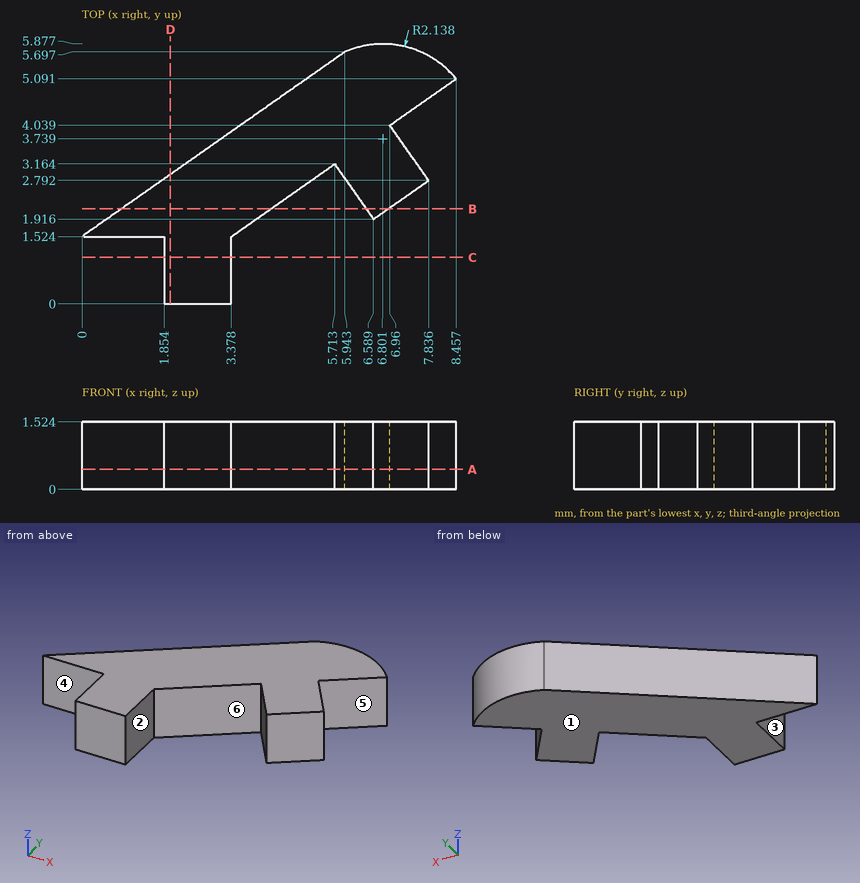
Could you check a few things on this drawing? It's one solid part, dimensions in mm from its lowest x, y, z. A direction names the side the tool comes from. Coordinates: 2 decimals unless noted, no trailing zeros. Order: outer loops, then holes, each group sorted by start corner. A loop starts at its lowest first (then second) coordinate and runs counter-clockwise, first axis right, second up. Notation, with made-up numbers: M -25.5,16 L -12.5,16 A26 ccw -12.5,36 Z; hole C 9.25,-6 d4. An arc over 180 degrees is marked long. Use a Markdown table: item, result. Add a question column.
Q1. I'm going to push flat-ended pins straight in: pin 1 (0.5 mm diameter, centred on x = 1, z = 0.5, fed in from -Y); pin 2 (0.8 mm diameter, centred on y = 1, z = 1, fed in from +X). Where does each tip first touch, or does it pass through?
Q2. I want a section at C-C on y = 1.05. List the corners of the cut face in (x, z) for me.
Q3. We'd pull the mould along X, two halves only. Please class the marked faces 4, 5 and 6: pulls with the +X half, pulls with the -X half, needs draft (parallel to the pull), parting line crosses it, or undercut.
Q4. I want a section at B-B on y = 2.15. List the corners of the cut face in (x, z) for me (1 decimal).
Q5. I want a section at A-A on z = 0.45. List the corners of the cut face in (x, y) for me (1 decimal).
Q6. Which directions (+Z, -Z, +X, -X, +Y, -Y) give clear straight access to the entire face, cutting with the end or side of a thin tool? Please do the marked faces 1, 2 and 3.
Q7. I want a section at D-D on x = 2. List the corners of the cut face in (y, z) for me.
Q8. If I drill on L1, parallel to X at y = 1.05, z = 1.4; L2, parallel to Y at x = 7.25, z = 0.25 (1 decimal); L3, parallel to X at y = 2.3, z = 0.7 (1 decimal), over which ranges is the centre line in solid material (lowest first)?
Checked values:
| question | item | result |
|---|---|---|
| 1 | pin 1 | y = 1.52 |
| 1 | pin 2 | x = 3.38 |
| 2 | outline | M 1.85,0 L 3.38,0 L 3.38,1.52 L 1.85,1.52 Z |
| 3 | face 4 | needs draft |
| 3 | face 5 | pulls with the +X half |
| 3 | face 6 | undercut |
| 4 | outline | M 0.9,0 L 4.3,0 L 4.3,1.5 L 0.9,1.5 Z; M 6.4,0 L 6.9,0 L 6.9,1.5 L 6.4,1.5 Z |
| 5 | outline | M 0,1.5 L 1.9,1.5 L 1.9,0 L 3.4,0 L 3.4,1.5 L 5.7,3.2 L 6.6,1.9 L 7.8,2.8 L 7,4 L 8.5,5.1 A2.1 ccw 5.9,5.7 Z |
| 6 | face 1 | -Z, +X, -X, +Y, -Y |
| 6 | face 2 | +Z, -Z, +X, -Y |
| 6 | face 3 | +Z, -Z, -X, -Y |
| 7 | outline | M 0,0 L 2.93,0 L 2.93,1.52 L 0,1.52 Z |
| 8 | L1 | 1.85 to 3.38 |
| 8 | L2 | 2.4 to 3.6, 4.2 to 5.8 |
| 8 | L3 | 1.1 to 4.5, 6.3 to 7.1 |
